Can you work these out from the model? Positions are in its coordinate system, mm. A direction names the side the tool comes from. Coordinates: 2 decimals unless noted, no trailing zeros. Loops run counter-clockwise (first coordinate to the right, second up) from the corner with the lowest first, then second, coordinate; pieces in that order, holes last.
```python
from build123d import *

# Parameters (mm, degrees)
PAD_DEPTH       = 2
SKETCH001_W     = 0.5
SKETCH001_H     = 4
PAD001_DEPTH    = 0.75
SKETCH002_W     = 0.5
SKETCH002_H     = 10
POCKET_DEPTH    = 1
SKETCH003_W     = 0.5
SKETCH003_H     = 0.5
POCKET001_DEPTH = 1
SKETCH004_W     = 0.5
SKETCH004_H     = 5
POCKET002_DEPTH = 0.5


with BuildPart() as part:
    # Sketch → Pad (new body)
    with BuildSketch(Plane.XY):
        Polygon((-4, 8), (4, 8), (4, 0), (7.5, -3), (7.5, -7), (-7.5, -7), (-7.5, -3), (-4, 0), align=None)
    extrude(amount=PAD_DEPTH)

    # Sketch001 (on Face9 of Pad) → Pad001 (join)
    with BuildSketch(Plane(origin=(0, 0, 0), x_dir=(1, 0, 0), z_dir=(0, 0, -1))):
        with Locations((0.875, -6)):
            Rectangle(SKETCH001_W, SKETCH001_H)
    extrude(amount=PAD001_DEPTH)

    # Sketch002 (on Face4 of Pad001) → Pocket (cut)
    with BuildSketch(Plane(origin=(0, 0, 0), x_dir=(1, 0, 0), z_dir=(0, 0, -1))):
        with Locations((-2.75, -3)):
            Rectangle(SKETCH002_W, SKETCH002_H)
        with Locations((-1.75, -3)):
            Rectangle(SKETCH002_W, SKETCH002_H)
        with Locations((-0.75, -3)):
            Rectangle(SKETCH002_W, SKETCH002_H)
        with Locations((2, -3)):
            Rectangle(SKETCH002_W, SKETCH002_H)
    extrude(amount=-POCKET_DEPTH, mode=Mode.SUBTRACT)

    # Sketch003 (on Sketch) → Pocket001 (cut)
    with BuildSketch(Plane.XY.offset(2)):
        with Locations((-2.75, -1.75)):
            Rectangle(SKETCH003_W, SKETCH003_H)
        with Locations((-1.75, -1.770407)):
            Rectangle(SKETCH003_W, SKETCH003_H)
        with Locations((-0.75, -1.75)):
            Rectangle(SKETCH003_W, SKETCH003_H)
        with Locations((2, -1.777476)):
            Rectangle(SKETCH003_W, SKETCH003_H)
    extrude(amount=-POCKET001_DEPTH, mode=Mode.SUBTRACT)

    # Sketch004 (on Face5 of Pocket001) → Pocket002 (cut)
    with BuildSketch(Plane.XY.offset(2)):
        with Locations((-2.75, -4.5)):
            Rectangle(SKETCH004_W, SKETCH004_H)
        with Locations((-1.75, -4.5)):
            Rectangle(SKETCH004_W, SKETCH004_H)
        with Locations((-0.75, -4.5)):
            Rectangle(SKETCH004_W, SKETCH004_H)
        with Locations((2, -4.5)):
            Rectangle(SKETCH004_W, SKETCH004_H)
    extrude(amount=-POCKET002_DEPTH, mode=Mode.SUBTRACT)


solid = part.part
```
Item 1: I need wall thicknesses on line 1 along X through (y, z) = (5.25, 0.2); line 2 along X through (y, z) = (-5.75, 1.6); line 3 along X through (y, z) = (3.5, 1.7). Which ranges of each line are inside material? Lowest first, please.
Results are:
line 1: x = -4 to -3, -2.5 to -2, -1.5 to -1, -0.5 to 1.75, 2.25 to 4
line 2: x = -7.5 to -3, -2.5 to -2, -1.5 to -1, -0.5 to 1.75, 2.25 to 7.5
line 3: x = -4 to 4
Item 2: Suppose I cut it at C-C, the plane x = -5.75. Please give me the cut outline in (y, z).
Results are:
outline: (-7, 0) - (-1.5, 0) - (-1.5, 2) - (-7, 2) - close
Item 3: I'm going to push flat-ended pins straight in: P1, Ø1, axis at y = 2, z = 0.5, coming from the +X side; P2, Ø1, axis at y = 6, z = 0.5, coming from the -X side; P3, Ø0.6, axis at y = -2.5, z = 0.5, coming from the +X side. Where does each tip first touch, or does it pass through?
Results are:
P1: stops at x = 4
P2: stops at x = -4
P3: stops at x = 7.27
Item 4: Suppose I cut it at A-A, the plane y = 1. Please give me the cut outline in (x, z), plus the area to 3 significant figures.
Results are:
outline: (-4, 0) - (-3, 0) - (-3, 1) - (-2.5, 1) - (-2.5, 0) - (-2, 0) - (-2, 1) - (-1.5, 1) - (-1.5, 0) - (-1, 0) - (-1, 1) - (-0.5, 1) - (-0.5, 0) - (1.75, 0) - (1.75, 1) - (2.25, 1) - (2.25, 0) - (4, 0) - (4, 2) - (-4, 2) - close
area: 14.0 mm2
Item 5: Suppose I cut it at D-D, the plane y = 4.75. Please give me the cut outline in (x, z) (3 decimals), plus the area to 3 significant figures.
Results are:
outline: (-4, 0) - (-3, 0) - (-3, 1) - (-2.5, 1) - (-2.5, 0) - (-2, 0) - (-2, 1) - (-1.5, 1) - (-1.5, 0) - (-1, 0) - (-1, 1) - (-0.5, 1) - (-0.5, 0) - (0.625, 0) - (0.625, -0.75) - (1.125, -0.75) - (1.125, 0) - (1.75, 0) - (1.75, 1) - (2.25, 1) - (2.25, 0) - (4, 0) - (4, 2) - (-4, 2) - close
area: 14.4 mm2
Item 6: On a 3-axis mill with a long thin cutter (end or side, diameter ignored), from which of +Z, -Z, +X, -X, +Y, -Y can I reach the whole of each face in a straight line? I mean faces 1 (the face through (-0.5, 2.3, 0.8)), 2 (the face through (0, 8, 1)), 3 (the face through (-4, 4, 1)), 4 (the face through (4, 4, 1)). Say none if no direction works.
Results are:
face 1: none
face 2: +Z, -Z, +X, -X, +Y
face 3: +Z, -Z, -X, +Y
face 4: +Z, -Z, +X, +Y
Item 7: Suppose I cut it at B-B, the plane z = 0.35. Please give me the cut outline in (x, y).
Results are:
outline: (-7.5, -7) - (7.5, -7) - (7.5, -3) - (4, 0) - (4, 8) - (2.25, 8) - (2.25, -2) - (1.75, -2) - (1.75, 8) - (-0.5, 8) - (-0.5, -2) - (-1, -2) - (-1, 8) - (-1.5, 8) - (-1.5, -2) - (-2, -2) - (-2, 8) - (-2.5, 8) - (-2.5, -2) - (-3, -2) - (-3, 8) - (-4, 8) - (-4, 0) - (-7.5, -3) - close
Item 8: We'd pull the mould along X, two halves only. Please class faces 5 (the face through (-2.5, 2.3, 0.8)), 6 (the face through (-5.774, -1.521, 0.986)), 7 (the face through (5.726, -1.479, 0.986)), 8 (the face through (-1.5, 2.3, 0.8)): +X half, -X half, draft (parallel to the pull), parting line (faces both ways), or undercut.
Results are:
face 5: undercut
face 6: -X half
face 7: +X half
face 8: undercut
